Autodesk Fusion 360 part; units mm, degrees
box "BoxPrimitive1" add length 38.0931 width 38.1 height 20.6375 placed x (0, -1, 0) y (1, 0, 0) z (0, 0, 1) at (0, 0, 0)
cylinder "CylinderPrimitive1" add diameter 29.3624 height 19.05 placed x (1, 0, 0) y (0, 1, 0) z (0, 0, 1) at (19.8488, -19.0466, 20.6375)
hole "Hole1" at (19.8488, -19.0466, 39.6875) direction (0, 0, -1) diameter 12.7 depth 35.2044 tip angle 180
hole "Hole2" at (38.1, -19.7481, 10.9094) direction (-1, 0, 0) diameter 11.1201 depth 18.1864 tip angle 180
Design review of the part built by this model. Coordinates are the model's own, in mm. A direction names the side the tool comes from. Coordinates: 2 decimals unless noted, no trailing zeros. Loops run counter-clockwise (first coordinate to the right, second up) from the corner with the lowest first, then second, coordinate; pieces in that order, holes last.
Item 1: Add section B-B (x = 11.5). Write out the cut boundary in (y, z), and give its area (3 significant figures).
Completed:
outline: (-38.09, 0) - (0, 0) - (0, 20.64) - (-6.97, 20.64) - (-6.97, 39.69) - (-31.12, 39.69) - (-31.12, 20.64) - (-38.09, 20.64) - close
area: 1,250 mm2
Item 2: For faces 1 (the cylindrical face through (31.29, -25.26, 11.63)), 2 (the cylindrical face through (27.741, -6.667, 30.296)), 3 (the flat face through (38.1, -15, 6)), list the 3-axis set-ups (+Z, -Z, +X, -X, +Y, -Y) from which the entire face can be reached by the end or side of a thin tool; tool diameter is ignored.
Completed:
face 1: +X
face 2: +Z
face 3: +Z, -Z, +X, +Y, -Y
Item 3: Add section A-A (y = -18). Write out the cut boundary in (x, z).
Completed:
outline: (0, 0) - (38.1, 0) - (38.1, 5.63) - (26.11, 5.63) - (26.11, 4.48) - (13.59, 4.48) - (13.59, 39.69) - (5.2, 39.69) - (5.2, 20.64) - (0, 20.64) - close; (26.11, 16.19) - (38.1, 16.19) - (38.1, 20.64) - (34.49, 20.64) - (34.49, 39.69) - (26.11, 39.69) - close
Item 4: Add section C-C (y = -5). Write out the cut boundary in (x, z).
Completed:
outline: (0, 0) - (38.1, 0) - (38.1, 20.64) - (24.12, 20.64) - (24.12, 39.69) - (15.58, 39.69) - (15.58, 20.64) - (0, 20.64) - close
Item 5: Add section D-D (z = 29). Write out the cut boundary in (x, y), and give its area (3 significant figures).
Completed:
outline: circle Ø29.36 at (19.85, -19.05); hole circle Ø12.7 at (19.85, -19.05)
area: 550 mm2
Item 6: Wall thickness on L1, parallel to Z at x = 36, y = -32; L2, parallel to Y at x = 17.5, z = 14.5; L3, parallel to Z at x = 17, y = -13.5: over which ranges is each line inside the solid? List them lowest first.
Completed:
L1: z = 0 to 20.64
L2: y = -38.09 to -24.95, -13.15 to 0
L3: z = 0 to 4.48
Item 7: Clearance check with flat-ended pins moving along their axes: pin 1 (8 mm diameter, centred on y = -22.5, z = 32, fed in from -X); pin 2 (4 mm diameter, centred on x = 18, y = -19, fed in from +Z); pin 3 (8 mm diameter, centred on y = -28.5, z = 28.5, fed in from -X). State where each tip first meets the part, or that it passes through.
Completed:
pin 1: stops at x = 5.17
pin 2: stops at z = 4.48
pin 3: stops at x = 6.22
Item 8: Draft analysis for pull direction X (two halves, no side actions). For faces 4 (the flat face through (0, -19, 10)), 5 (the cylindrical face through (13.553, -18.22, 21.839)), 6 (the flat face through (20, -19, 4.483)), 7 (the flat face through (19, 0, 10)), state which applies: pulls with the +X half, pulls with the -X half, needs draft (parallel to the pull), parting line crosses it, or undercut.
Completed:
face 4: pulls with the -X half
face 5: undercut
face 6: undercut
face 7: needs draft
